Here's how the part is built. I have some questions about the finished solid (model axes, mm). Face numbers are marked on the shaded views. A direction names the side the tool comes from. Give positions to 0.01 mm unless a question says otherwise; leave off trailing zeros. Write each loop counter-clockwise with the first axis right and the second up, starting at its lowest first coordinate (ties: lowest second). Pieces come first, ordered by that corner, then holes. Notation, with made-up numbers: M -35.5,20.25 L 18.5,20.25 A22 ccw 18.5,39.25 Z; hole C -1,3.5 d7. An arc over 180 degrees is marked long. Use one line per item in the form item = value. Start each with the question number.
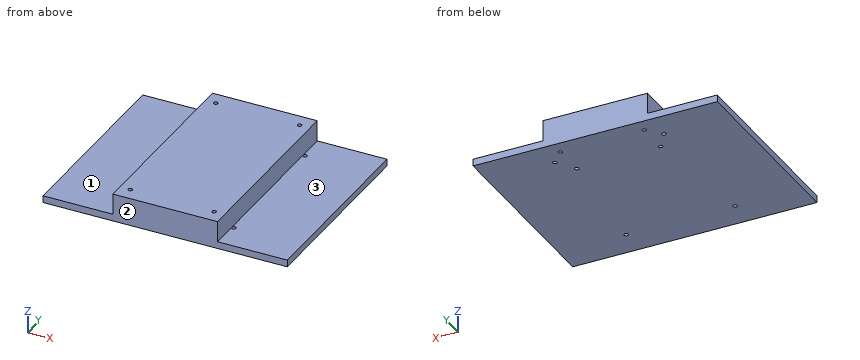
Autodesk Fusion 360 part; units mm, degrees
sketch "Sketch1" plane through (0, 0, 0) normal (0, 0, 1) x (1, 0, 0)
  line L0 (0, 0) -> (175, 0)
  line L1 (175, 0) -> (175, 140)
  line L2 (175, 140) -> (0, 140)
  line L3 (0, 140) -> (0, 0)
  line L4 (50, 140) -> (50, 0)
  line L5 (125, 140) -> (125, 0)
  circle A0 centre (57.5, 10) radius 1.5
  circle A1 centre (117.5, 10) radius 1.5
  line L6 (87.5, 0) -> (87.5, 140) construction
  circle A2 centre (57.5, 130) radius 1.5
  circle A3 centre (117.5, 130) radius 1.5
  line L7 (57.5, 130) -> (57.5, 100) construction
  circle A4 centre (57.5, 107) radius 1.5
  line L8 (117.5, 130) -> (117.5, 100) construction
  circle A5 centre (117.5, 107) radius 1.5
  circle A6 centre (48.5, 120) radius 1.5
  line L9 (0, 70) -> (175, 70) construction
  circle A7 centre (48.5, 20) radius 1.5
  circle A8 centre (126.5, 120) radius 1.5
  circle A9 centre (126.5, 20) radius 1.5
  dimension "d1" = 140
  dimension "d2" = 175
  dimension "d3" = 50
  dimension "d4" = 50
  dimension "d5" = 3
  dimension "d6" = 10
  dimension "d7" = 3
  dimension "d10" = 60
  dimension "d11" = 3
  dimension "d12" = 3
  dimension "d13" = 60
  dimension "d14" = 10
  dimension "d23" = 3
  dimension "d24" = 23
  dimension "d25" = 3
  dimension "d26" = 23
  dimension "d27" = 3
  dimension "d28" = 3
  dimension "d29" = 100
  dimension "d30" = 3
  dimension "d31" = 3
  dimension "d32" = 100
extrude "Extrude1" add sketch "Sketch1" along normal blind 20 contours L0 L2 L4 L5
extrude "Extrude3" add sketch "Sketch1" along normal blind 5 contours L0 L2 L3 L4 | L0 L1 L2 L5
extrude "Extrude4" add sketch "Sketch1" along normal blind 15 contours A0 | A1
extrude "Extrude5" add sketch "Sketch1" along normal blind 10 from surface at 5 contours A2 | A3
extrude "Extrude6" add sketch "Sketch1" along normal blind 15 from surface at 5 contours A4 | A5
1) Will these pins go through, and if not, where does the flat tip stop? P1, Ø2, axis at y = 104, z = 15, coming from the +X side; P2, Ø5, axis at x = 142, y = 82, coming from the +Z side; P3, Ø0.9, axis at x = 117.5, y = 107, coming from the -Z side.
2) Suppose I cut it at B-B, the plane z = 9. List the corners of the cut face in (x, y) for me.
3) On a 3-axis mill with a long thin cutter (end or side, diameter ignored), from which of +Z, -Z, +X, -X, +Y, -Y can I reach the whole of each face in a straight line? I mean the marked faces 1, 2 and 3. Say none if no direction works.
4) Suppose I cut it at A-A, the plane x = 40. List the corners of the cut face in (y, z) for me.
5) Please list where these lines run through material, in increasing order: line 1 (Y direction, x = 117.5, z = 16.2); line 2 (Y direction, x = 126.5, z = 1.5); line 3 (X direction, y = 120, z = 2.45).
Checks:
q1.P1 = 125
q1.P2 = 5
q1.P3 = 5
q2.outline = M 50,0 L 125,0 L 125,140 L 50,140 Z
q3.face_1 = +Z, -X, +Y, -Y
q3.face_2 = +Z, -Z, +X, -X, -Y
q3.face_3 = +Z, +X, +Y, -Y
q4.outline = M 0,0 L 140,0 L 140,5 L 0,5 Z
q5.line_1 = 0 to 8.5, 11.5 to 128.5, 131.5 to 140
q5.line_2 = 0 to 18.5, 21.5 to 118.5, 121.5 to 140
q5.line_3 = 0 to 47, 50 to 125, 128 to 175
